Autodesk Inventor part; units mm, degrees
ref_plane "YZ Plane" through (0, 0, 0) normal (1, 0, 0) x (0, 1, 0)
ref_plane "XZ Plane" through (0, 0, 0) normal (0, 1, 0) x (-1, 0, 0)
ref_plane "XY Plane" through (0, 0, 0) normal (0, 0, 1) x (1, 0, 0)
sketch "Sketch1" plane through (0, 0, 0) normal (0, 1, 0) x (-1, 0, 0)
  line L0 (-143.1635, -20.2145) -> (110.8365, -20.2145)
  line L1 (110.8365, -20.2145) -> (110.8365, -52.2145)
  line L2 (110.8365, -52.2145) -> (-143.1635, -52.2145)
  line L3 (-143.1635, -52.2145) -> (-143.1635, -20.2145)
  circle A0 centre (-16.1635, -36.2145) radius 8
  point P0 (0, 0)
  dimension "d0" = 254
  dimension "d1" = 32
  dimension "d10" = 16
  dimension "d11" = 127
  dimension "d12" = 16
extrude "Extrusion1" add sketch "Sketch1" along normal blind 1
chamfer "Chamfer1" distance 100 distance2 1 1 edges at (143.1635, 1, -36.2145) measured on face at (103.4969, 1, -36.2145)
chamfer "Chamfer2" distance 100 distance2 1 1 edges at (-110.8365, 1, -36.2145) measured on face at (-71.1698, 1, -36.2145)
properties part number "lama"
Work out the finished part from the listing and answer in its coordinate system (mm). Coordinates: 2 decimals unless noted, no trailing zeros. Loops run counter-clockwise (first coordinate to the right, second up) from the corner with the lowest first, then second, coordinate; pieces in that order, holes last. Notation, with made-up numbers: M -15,-34 L 38,-34 A11 ccw 38,-21 Z; hole C 40.5,63 d5. An arc over 180 degrees is marked long. Use CSV: the item, a comma, the result in double quotes. Start each with the question number.
(1) Consider line 1 (Y direction, x = 126.5, z = -24); line 2 (Y direction, x = -26.5, z = -49.5); line 3 (Z direction, x = 19, y = 0.2). Determine where each line is inside the solid, lowest interval first.
(2) Find section C-C, the plane x = 18.5. Give the vertices of the cut face in (y, z).
(3) Find section D-D, the plane x = 95.5. Give the vertices of the cut face in (y, z), then the cut area to 3 significant figures.
(4) Find section B-B, the plane y = 0.65. Give the vertices of the cut face in (x, z).
(5) For a pull along Z with two mould halves and no side action, classify faces 1 (the face through (18, 0, -25)), 2 (the face through (17.898, 0.493, -28.405)) as +Z half, -Z half, draft (parallel to the pull), parting line (faces both ways), or undercut.
(6) Given pin 1 Ø18.5 at (x, z) = (16.16, -36.21) entering from -Y; pin 2 Ø10 at (x, z) = (-34.5, -28) entering from +Y, each flat-ended and moving along its own axis, determine where each tip first touches the part or whether it passes through.
Recorded:
1,line 1,"y = 0 to 0.17"
1,line 2,"y = 0 to 0.84"
1,line 3,"z = -52.21 to -43.69, -28.73 to -20.21"
2,outline,"M 0,-52.21 L 1,-52.21 L 1,-43.87 L 0,-43.87 Z; M 0,-28.56 L 1,-28.56 L 1,-20.21 L 0,-20.21 Z"
3,outline,"M 0,-52.21 L 0.48,-52.21 L 0.48,-20.21 L 0,-20.21 Z"
3,area,"15.3 mm^2"
4,outline,"M -45.85,-52.21 L 78.18,-52.21 L 78.18,-20.21 L -45.85,-20.21 Z; hole C 16.16,-36.21 d16"
5,face 1,"draft"
5,face 2,"undercut"
6,pin 1,"stops at y = 0"
6,pin 2,"stops at y = 0.81"
